from build123d import *

# Parameters (mm, degrees)
SKETCH1_R             = 15
BOSS_EXTRUDE1_DEPTH   = 10
BOSS_EXTRUDE1_2_DEPTH = 10
SKETCH2_R             = 15
BOSS_EXTRUDE2_DEPTH   = 10
BOSS_EXTRUDE2_TAPER   = 20
BOSS_EXTRUDE3_DEPTH   = 5
BOSS_EXTRUDE4_DEPTH   = 5
SKETCH13_R            = 4
CUT_EXTRUDE1_DEPTH    = 20
BOSS_EXTRUDE7_START   = 2.5
SKETCH14_R            = 15
SKETCH14_R_2          = 4
BOSS_EXTRUDE7_DEPTH   = 2.5


with BuildPart() as part:
    # Sketch1 → Boss-Extrude1 (new body)
    with BuildSketch(Plane.XY):
        Circle(SKETCH1_R)
    extrude(amount=BOSS_EXTRUDE1_DEPTH)

    # Sketch2 → Boss-Extrude2 (add)
    with BuildSketch(Plane.XY.offset(10)):
        Circle(SKETCH2_R)
    extrude(amount=BOSS_EXTRUDE2_DEPTH, taper=BOSS_EXTRUDE2_TAPER)



with BuildPart() as body_2:
    # Sketch1 → Boss-Extrude1 2 (new body)
    with BuildSketch(Plane.XY):
        with Locations((215, 0)):
            Circle(SKETCH1_R)
    extrude(amount=BOSS_EXTRUDE1_2_DEPTH)


with BuildPart() as part_1:
    add(part.part)

    add(body_2.part)  # Boss-Extrude3 merges body 2
    # Sketch5 → Boss-Extrude3 (add)
    with BuildSketch(Plane.XY):
        with BuildLine():
            Line((203.819660113, 10), (11.180339887, 10))
            ThreePointArc((11.180339887, 10), (14.012585384, 5.352331347), (15, 0))
            ThreePointArc((15, 0), (14.012585384, -5.352331347), (11.180339887, -10))
            Line((11.180339887, -10), (203.819660113, -10))
            ThreePointArc((203.819660113, -10), (200, 0), (203.819660113, 10))
        make_face()
    extrude(amount=BOSS_EXTRUDE3_DEPTH)

    # Sketch6 → Boss-Extrude4 (add)
    with BuildSketch(Plane.XY.offset(5)):
        with BuildLine():
            ThreePointArc((15, 0), (14.947457842, -1.254393904), (14.790199458, -2.5))
            ThreePointArc((14.790199458, -2.5), (13.515906498, -6.505403256), (11.180339887, -10))
            Line((11.180339887, -10), (203.819660113, -10))
            ThreePointArc((203.819660113, -10), (200, 0), (203.819660113, 10))
            Line((203.819660113, 10), (11.180339887, 10))
            ThreePointArc((11.180339887, 10), (13.515906498, 6.505403256), (14.790199458, 2.5))
            ThreePointArc((14.790199458, 2.5), (14.947457842, 1.254393904), (15, 0))
        make_face()
    extrude(amount=BOSS_EXTRUDE4_DEPTH)

    # Sketch13 → Cut-Extrude1 (cut)
    with BuildSketch(Plane(origin=(0, 0, 0), x_dir=(-1, 0, 0), z_dir=(0, 0, -1))):
        with Locations((-215, 0)):
            Circle(SKETCH13_R)
        Circle(SKETCH13_R)
    extrude(amount=-CUT_EXTRUDE1_DEPTH, mode=Mode.SUBTRACT)

    # Sketch14 → Boss-Extrude7 (add)
    with BuildSketch(Plane(origin=(0, 0, 0), x_dir=(-1, 0, 0), z_dir=(0, 0, -1)).offset(BOSS_EXTRUDE7_START)):
        Circle(SKETCH14_R)
        Circle(SKETCH14_R_2, mode=Mode.SUBTRACT)
    extrude(amount=-BOSS_EXTRUDE7_DEPTH)


solid = part_1.part
Input: part model. Units: mm. Frame: model coordinates. A direction names the side the tool comes from. Round coordinates to 2 decimals unless told otherwise and drop trailing zeros. Write each loop counter-clockwise with the first axis right and the second up, starting at its lowest first coordinate (ties: lowest second). Pieces come first, ordered by that corner, then holes.
1) Cut plane A-A (x = 0). Return the cut outline in (y, z).
2) Ray query, L1, parallel to X at y = -0.5, z = -0.5; L2, parallel to X at y = 0.75, z = 2.5; L3, parallel to X at y = -1.75, z = 2.25. Return the intervals inside material, ascending.
3) Cut plane D-D (x = 215). Return the cut outline in (y, z), then the cut area to 3 significant figures.
4) Cut plane B-B (y = 0). Return the cut outline in (x, z), then the cut area to 3 significant figures.
5) Cut plane C-C (z = 2.25). Return the cut outline in (x, y).
6) Reachability of faces 4 (the cylindrical face through (229.99, -0.51, 4.93)), 5 (the flat face through (106, -10, 5)), 6 (the flat face through (109, 10, 5)) from +Z, -Z, +X, -X, +Y, -Y: full face, straight path, thin tool, end or side. Return the list, or none.
7) Contact query for flat-ended pins moving along their axis: P1, Ø12, axis at y = -12, z = 7, coming from the +X side; P2, Ø5, axis at x = 215, y = 0, coming from the +Z side; P3, Ø12, axis at x = 106, z = 11, coming from the +Y side; P4, Ø5, axis at x = 40, z = 0, coming from the -Y side. Output: stop coordinate, or through.
8) Draft query along X for faces 1 (the flat face through (5, 0, 20)), 2 (the conical face through (-1.5, 11.44, 19.51)), 3 (the cylindrical face through (219, 0, 5)). Return one class per face: pulls with the +X half, pulls with the -X half, needs draft (parallel to the pull), parting line crosses it, or undercut.
Geometry says:
1. outline: (-15, -2.5) - (-4, -2.5) - (-4, 20) - (-11.36, 20) - (-15, 10) - close; (4, -2.5) - (15, -2.5) - (15, 10) - (11.36, 20) - (4, 20) - close
2. L1: x = -14.99 to -3.97, 3.97 to 14.99
2. L2: x = -14.98 to -3.93, 3.93 to 211.07, 218.93 to 229.98
2. L3: x = -14.9 to -3.6, 3.6 to 211.4, 218.6 to 229.9
3. outline: (-15, 0) - (-4, 0) - (-4, 10) - (-15, 10) - close; (4, 0) - (15, 0) - (15, 10) - (4, 10) - close
3. area: 220 mm2
4. outline: (-15, -2.5) - (-4, -2.5) - (-4, 20) - (-11.36, 20) - (-15, 10) - close; (4, -2.5) - (15, -2.5) - (15, 0) - (211, 0) - (211, 10) - (15, 10) - (11.36, 20) - (4, 20) - close; (219, 0) - (230, 0) - (230, 10) - (219, 10) - close
4. area: 2,530 mm2
5. outline: (11.18, -10) - (203.82, -10) arc R15 ccw (long way) to (203.82, 10) - (11.18, 10) arc R15 ccw (long way) to start; hole circle Ø8 at (0, 0); hole circle Ø8 at (215, 0)
6. face 4: +Z, -Z
6. face 5: +Z, -Z, -Y
6. face 6: +Z, -Z, +Y
7. P1: stops at x = 228.75
7. P2: passes through
7. P3: stops at y = 10
7. P4: stops at y = -10
8. face 1: needs draft
8. face 2: parting line crosses it
8. face 3: undercut
